Input: part model. Units: mm. Frame: model coordinates. A direction names the side the tool comes from. Round coordinates to 2 decimals unless told otherwise and drop trailing zeros. Order: outer loops, then holes, each group sorted by start corner. A loop starts at its lowest first (then second) coordinate and runs counter-clockwise, first axis right, second up. Notation, with made-up numbers: (28.5, 61) -> (69.5, 61) arc R21 cw to (69.5, 90) -> close; hole circle Ø11 at (-2, -21). An arc over 180 degrees is marked (long way). Use a Markdown table: item, result.
from build123d import *

# Parameters (mm, degrees)
CYLINDER011_R     = 2.85
CYLINDER011_DEPTH = 3.1
CYLINDER010_R     = 1.6
CYLINDER010_DEPTH = 4.5
CYLINDER001_R     = 3
CYLINDER001_DEPTH = 1
EXTRUDE001_DEPTH  = 3.5


with BuildPart() as bearingbracket_m3head:
    # Cylinder011 → Cylinder011 (new body)
    with BuildSketch(Plane.XZ):
        Circle(CYLINDER011_R)
    extrude(amount=CYLINDER011_DEPTH)


with BuildPart() as bearingbracket_m3cutout:
    # Cylinder010 → Cylinder010 (new body)
    with BuildSketch(Plane.XZ):
        Circle(CYLINDER010_R)
    extrude(amount=CYLINDER010_DEPTH)

    # Fusion: union bearingBracket_m3Head
    add(bearingbracket_m3head.part)


with BuildPart() as bearingbracket_m3cutout_1:
    # Fusion placement: moved
    add(bearingbracket_m3cutout.part.moved(Location((0, 3.5, 0))))


with BuildPart() as bearingbracket_spacer:
    # Cylinder001 → Cylinder001 (new body)
    with BuildSketch(Plane.XZ):
        Circle(CYLINDER001_R)
    extrude(amount=CYLINDER001_DEPTH)


with BuildPart() as bearingbracket:
    # Sketch001 → Extrude001 (new body)
    with BuildSketch(Plane.XZ):
        with BuildLine():
            ThreePointArc((-4.46354, -1.624596), (0, -4.75), (4.46354, -1.624596))
            Line((4.46354, -1.624596), (5.054844, 0))
            Line((5.054844, 0), (7.056681, 5.5))
            Line((-7.056681, 5.5), (7.056681, 5.5))
            Line((-5.054844, 0), (-7.056681, 5.5))
            Line((-4.46354, -1.624596), (-5.054844, 0))
        make_face()
    extrude(amount=-EXTRUDE001_DEPTH)

    # Fusion001: union bearingBracket_spacer
    add(bearingbracket_spacer.part)

    # Cut011: cut bearingBracket_m3Cutout
    add(bearingbracket_m3cutout_1.part, mode=Mode.SUBTRACT)


with BuildPart() as bearingbracket_1:
    # Cut011 placement: moved
    add(bearingbracket.part.moved(Location((0, 41.5, 0))))


solid = bearingbracket_1.part
1) Set-up query: faces 4 (the cylindrical face through (-2.262, 43.472, -1.734)), 5 (the flat face through (1.3, 40.5, -1.3)). Return all of +Z, -Z, +X, -X, +Y, -Y with unobstructed straight access to the full face (end or side cutting, diameter ignored); none if empty.
Results found:
| item | result |
|---|---|
| face 4 | +Y |
| face 5 | +Z, -Z, +X, -X, -Y |
2) Cut plane C-C on z = 0.5. Return loops of the section in (x, y), and give its area (3 significant figures).
Results found:
| item | result |
|---|---|
| outline | (-5.24, 41.5) -> (-2.96, 41.5) -> (-2.96, 40.5) -> (-1.52, 40.5) -> (-1.52, 41.9) -> (-2.81, 41.9) -> (-2.81, 45) -> (-5.24, 45) -> close; (1.52, 40.5) -> (2.96, 40.5) -> (2.96, 41.5) -> (5.24, 41.5) -> (5.24, 45) -> (2.81, 45) -> (2.81, 41.9) -> (1.52, 41.9) -> close |
| area | 20.9 mm² |
3) Cut plane A-A on x = 0. Return loops of the section in (y, z).
Results found:
| item | result |
|---|---|
| outline | (40.5, -3) -> (41.5, -3) -> (41.5, -4.75) -> (45, -4.75) -> (45, -2.85) -> (41.9, -2.85) -> (41.9, -1.6) -> (40.5, -1.6) -> close; (40.5, 1.6) -> (41.9, 1.6) -> (41.9, 2.85) -> (45, 2.85) -> (45, 5.5) -> (41.5, 5.5) -> (41.5, 3) -> (40.5, 3) -> close |
4) Line query: L1, parallel to Z at x = 0, y = 44; L2, parallel to Z at x = 0, y = 41.35; L3, parallel to Y at x = 2, z = 1.25. Output: solid intervals per line, ascending. Write a range as [from, to].
Results found:
| item | result |
|---|---|
| L1 | z = [-4.75, -2.85], [2.85, 5.5] |
| L2 | z = [-3, -1.6], [1.6, 3] |
| L3 | y = [40.5, 41.9] |
5) Cut plane B-B on y = 43.75. Return loops of the section in (x, z).
Results found:
| item | result |
|---|---|
| outline | (-7.06, 5.5) -> (-5.05, 0) -> (-4.46, -1.62) arc R4.75 ccw to (4.46, -1.62) -> (5.05, 0) -> (7.06, 5.5) -> close; hole circle Ø5.7 at (0, 0) |
6) Pull-direction query (Z, two-part tool) for faces 1 (the cylindrical face through (-3, 41, 0)), 2 (the flat face through (1, 41.5, 3)), 3 (the cylindrical face through (-1.27, 41.21, -0.97)); classes: +Z half, -Z half, draft (parallel to the pull), parting line (faces both ways), or undercut.
Results found:
| item | result |
|---|---|
| face 1 | parting line |
| face 2 | draft |
| face 3 | undercut |
7) Cut plane D-D on z = 2. Return loops of the section in (x, y).
Results found:
| item | result |
|---|---|
| outline | (-5.78, 41.5) -> (-2.24, 41.5) -> (-2.24, 40.5) -> (2.24, 40.5) -> (2.24, 41.5) -> (5.78, 41.5) -> (5.78, 45) -> (2.03, 45) -> (2.03, 41.9) -> (-2.03, 41.9) -> (-2.03, 45) -> (-5.78, 45) -> close |
